from build123d import *

# Parameters (mm, degrees)
F0_W     = 120.65
F0_H     = 95.25
F0_W_2   = 101.6
F0_H_2   = 76.2
F1_DEPTH = 152.4
F2_W     = 9.525
F2_H     = 95.25
F3_DEPTH = 120.65
F4_W     = 120.65
F4_H     = 1.27
F5_DEPTH = 9.525
F6_W     = 8
F6_H     = 15
F6_R     = 2.5
F7_DEPTH = 25.4
F8_W     = 74.93
F8_H     = 1.27
F9_DEPTH = 179.07


with BuildPart() as f1:
    # F0 (on Front) → F1 (new body)
    with BuildSketch(Plane.XZ):
        with Locations((1.705641, 0)):
            Rectangle(F0_W, F0_H)
        with Locations((1.705641, 0)):
            Rectangle(F0_W_2, F0_H_2, mode=Mode.SUBTRACT)
    extrude(amount=F1_DEPTH)

    # F2 (on face) → F3 (join)
    with BuildSketch(Plane(origin=(-58.619359, 0, 0), x_dir=(0, -1, 0), z_dir=(-1, 0, 0))):
        with Locations((-4.7625, 0)):
            Rectangle(F2_W, F2_H)
        with Locations((157.1625, 0)):
            Rectangle(F2_W, F2_H)
    extrude(amount=-F3_DEPTH)

    # F4 (on face) → F5 (cut)
    with BuildSketch(Plane.XY.offset(47.625)):
        with Locations((1.705641, -76.835)):
            Rectangle(F4_W, F4_H)
    extrude(amount=-F5_DEPTH, mode=Mode.SUBTRACT)

    # F6 (on face) → F7 (cut)
    with BuildSketch(Plane.XY.offset(47.625)):
        with Locations((0, -42.425)):
            Rectangle(F6_W, F6_H)
        with Locations((-29.4, -42.425)):
            Circle(F6_R)
        with Locations((29.4, -42.425)):
            Circle(F6_R)
    extrude(amount=-F7_DEPTH, mode=Mode.SUBTRACT)

    # F8 (on face) → F9 (cut)
    with BuildSketch(Plane(origin=(-58.619359, 0, 0), x_dir=(0, -1, 0), z_dir=(-1, 0, 0))):
        with Locations((114.935, 38.735)):
            Rectangle(F8_W, F8_H)
    extrude(amount=-F9_DEPTH, mode=Mode.SUBTRACT)


solid = f1.part
Geometry check sheet. Reference: the model listing, model coordinates, mm. A direction names the side the tool comes from. Give positions to 0.01 mm unless a question says otherwise; leave off trailing zeros. Write each loop counter-clockwise with the first axis right and the second up, starting at its lowest first coordinate (ties: lowest second). Pieces come first, ordered by that corner, then holes. Notation, with made-up numbers: M 47,24.5 L 65,24.5 A15 ccw 65,31.5 Z; hole C 40.25,55.25 d10. An arc over 180 degrees is marked long. One line per question, with ' | ' between items.
1. Set-up check for faces 1 (the face through (-49.094, -75, -1)), 2 (the face through (0, -49.925, 43)), 3 (the face through (1, -114, 39.37)): record each of +Z, -Z, +X, -X, +Y, -Y from which the full face is reachable in a straight line by a thin tool's end or side.
Ans:
face 1: none | face 2: +Z | face 3: +X, -X
2. Cross-section at B-B (y = -150.5). Enter the section's corners in (x, z) (3 decimals).
Ans:
outline: M -58.619,-47.625 L 62.031,-47.625 L 62.031,38.1 L 52.506,38.1 L 52.506,-38.1 L -49.094,-38.1 L -49.094,38.1 L -58.619,38.1 Z; M -58.619,39.37 L 62.031,39.37 L 62.031,47.625 L -58.619,47.625 Z
3. Cross-section at A-A (x = -2). Enter the section's corners in (y, z) (3 decimals), plus the area to 3 significant figures.
Ans:
outline: M -161.925,-47.625 L 9.525,-47.625 L 9.525,47.625 L -34.925,47.625 L -34.925,38.1 L 0,38.1 L 0,-38.1 L -152.4,-38.1 L -152.4,39.37 L -77.47,39.37 L -77.47,47.625 L -161.925,47.625 Z; M -76.2,38.1 L -49.925,38.1 L -49.925,47.625 L -76.2,47.625 Z | area: 4,470 mm2
4. Mould release check, pull along X, two halves, no side actions. Record for faces 4 (the face through (62.031, -75, 1)), 5 (the face through (1, -76.2, 43)), 6 (the face through (-4, -43, 43)): released by +X, released by -X, zero draft, split by the parting line, or undercut.
Ans:
face 4: released by +X | face 5: zero draft | face 6: undercut
5. Cross-section at C-C (y = -57). Enter the section's corners in (x, z) (3 decimals), plus the area to 3 significant figures.
Ans:
outline: M -58.619,-47.625 L 62.031,-47.625 L 62.031,47.625 L -58.619,47.625 Z; hole M -49.094,-38.1 L 52.506,-38.1 L 52.506,38.1 L -49.094,38.1 Z | area: 3,750 mm2
6. Scan lines: line 1 along Y through (x, z) = (29, 40) (3 decimals); line 2 along Y through (x, z) = (33, -9.5) (3 decimals); line 3 along Z through (x, y) = (-19, -106.5) (3 decimals). Record each from-to range of solid material in increasing order. Write a range as from..to.
Ans:
line 1: -161.925..-77.47, -76.2..-44.893, -39.957..9.525 | line 2: -161.925..-152.4, 0..9.525 | line 3: -47.625..-38.1, 39.37..47.625
7. Cross-section at D-D (z = 33). Enter the section's corners in (x, y) (3 decimals), plus the area to 3 significant figures.
Ans:
outline: M -58.619,-161.925 L 62.031,-161.925 L 62.031,9.525 L -58.619,9.525 Z; hole M -49.094,-152.4 L 52.506,-152.4 L 52.506,0 L -49.094,0 Z | area: 5,200 mm2
8. Gauge pin test, flat end, axial feed: pin 1 (4.5 mm diameter, centred on x = 29.4, y = -42.425, fed in from +Z). Record the tip position at first contact, or that the pin passes through.
Ans:
pin 1: z = -38.1
